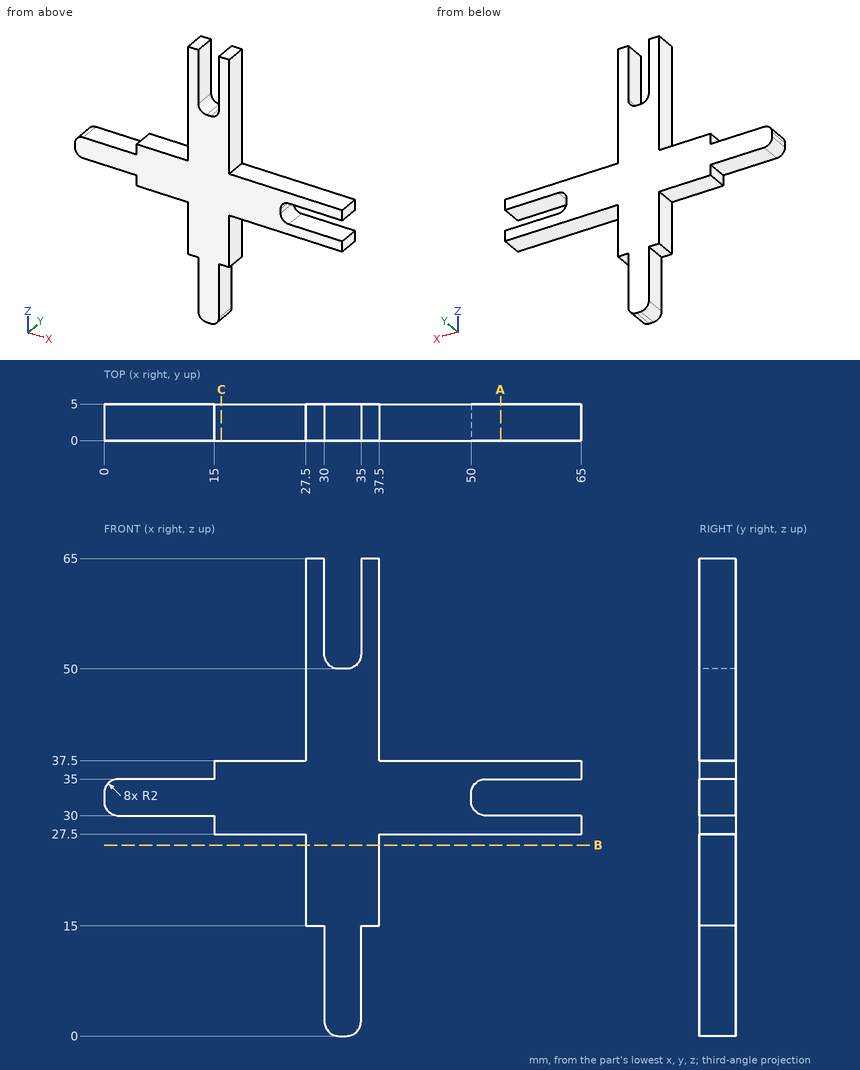
Could you check a few things on this drawing? It's one solid part, dimensions in mm from its lowest x, y, z. Coordinates: 2 decimals unless noted, no trailing zeros. Order: outer loops, then holes, each group sorted by start corner. A loop starts at its lowest first (then second) coordinate and runs counter-clockwise, first axis right, second up. Notation, with made-up numbers: M 27,-8 L 36,-8 A16 cw 36,14 Z; hole C -39,55 d11. An arc over 180 degrees is marked long. Answer as a JSON object with one key per item and string values. Group by question number.
(1) Suppose I cut it at B-B, the plane z = 26. Please give me the cut outline in (x, y), then the cut area to 3 significant figures.
(2) Suppose I cut it at C-C, the plane x = 16. Please give me the cut outline in (y, z).
(3) I need wall thicknesses on probe 1 along X at (y, z) = (3.35, 61); probe 2 along X at (y, z) = (4.65, 42.5). Which ranges of each line are inside material? Lowest first, please.
(4) Suppose I cut it at A-A, the plane x = 54. Please give me the cut outline in (y, z).
(5) For pin 1 (1.5 mm diameter, centred on x = 46.5, y = 2.5, fed in from +Z); pin 2 (1.5 mm diameter, centred on x = 24, y = 2, fed in from -Z); pin 3 (2 mm diameter, centred on y = 1.5, z = 18.5, fed in from -X), each with a flat end and sliding along its axis, tell me the tip position at first contact or that it passes through.
Values found:
{
 "1": {"outline": "M 27.5,0 L 37.5,0 L 37.5,5 L 27.5,5 Z", "area": "50.0 mm^2"},
 "2": {"outline": "M 0,27.5 L 5,27.5 L 5,37.5 L 0,37.5 Z"},
 "3": {"probe 1": "x = 27.5 to 30, 35 to 37.5", "probe 2": "x = 27.5 to 37.5"},
 "4": {"outline": "M 0,27.5 L 5,27.5 L 5,30 L 0,30 Z; M 0,35 L 5,35 L 5,37.5 L 0,37.5 Z"},
 "5": {"pin 1": "stops at z = 37.5", "pin 2": "stops at z = 27.5", "pin 3": "stops at x = 27.5"}
}
